Source: CAD feature listing. Evaluate the final solid. Frame: model axes, mm. Face numbers are marked on the shaded views. A direction names the side the tool comes from. Round coordinates to 2 decimals unless told otherwise and drop trailing zeros. Order: outer loops, then holes, each group sorted by start corner. A loop starts at its lowest first (then second) coordinate and runs counter-clockwise, first axis right, second up. Notation, with made-up numbers: (-13.75, 80) - (42.25, 80) arc R33 ccw to (42.25, 115) - close; hole circle Ø11 at (46.5, -8). An arc over 180 degrees is marked (long way). Return JSON: item names as keys, results as strings. Group by question number.
1) Section A-A, the plane z = 11.5. Return loops of the section in (x, y), plus the area to 3 significant figures.
2) Access query for the marked faces 3 and 4. Directions: +Z, -Z, +X, -X, +Y, -Y. A direction counts if a zero-diameter tool reaches every point of the face in a straight line with its end or side. Return the directions, or none.
3) Ray query, line 1 (X direction, y = 2, z = 17); line 2 (Z direction, x = -0.5, y = 4); line 3 (Z direction, x = 0.5, y = 0.5). Return the intervals inside material, ascending. Write a range as from..to.
4) Contact query for flat-ended pins moving along their axis: P1, Ø0.9, axis at x = 0, y = 0.5, coming from the +Z side; P2, Ø1, axis at y = -1, z = 26, coming from the -X side; P3, Ø1, axis at y = 0, z = 18, coming from the +X side. Output: stop coordinate, or through.
5) Mould query, pull axis X, two halves, no side actions, for the marked faces 1 and 2. Classes: pulls with the +X half, pulls with the -X half, needs draft (parallel to the pull), parting line crosses it, or undercut.
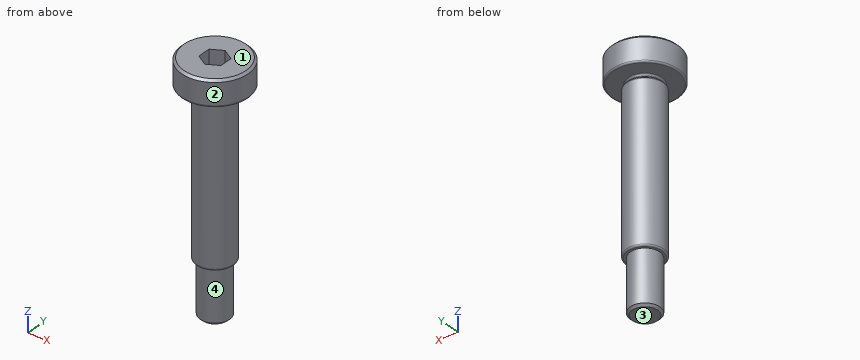
Solid Edge part; units mm, degrees
sketch "Sketch1" plane through (0, 0, 0) normal (0, -1, 0) x (1, 0, 0)
  line L0 (0, 32.7) -> (4.505, 32.7)
  line L1 (4.505, 32.7) -> (4.505, 29.25)
  line L2 (4.505, 29.25) -> (2.1, 29.25)
  line L3 (2.1, 29.25) -> (2.1, 28.85)
  line L4 (2.1, 28.85) -> (2.5, 28.85)
  line L5 (2.5, 28.85) -> (2.5, 7.25)
  line L6 (2.5, 7.25) -> (2, 7.25)
  line L7 (2, 7.25) -> (2, 0)
  line L8 (2, 0) -> (0, 0)
  dimension "D1" = 4.505
  dimension "D2" = 2.1
  dimension "D3" = 2
  dimension "D4" = 2.5
  dimension "D5" = 2
revolve "RevolvedProtrusion1" add sketch "Sketch1" angle 360 about axis through (0, 0, 0) along (0, 0, 1)
chamfer "Chamfer1" distance 0.3 angle 45 3 edges at (-2.5, 0, 28.85) (-4.505, 0, 32.7) (-2, 0, 0)
fillet "Round_1" radius 0.2 4 edges at (-4.505, 0, 29.25) (-2.1, 0, 29.25) (-2.5, 0, 7.25) (-2.5, 0, 28.55)
sketch "Sketch2" plane through (0, 0, 32.7) normal (0, 0, 1) x (1, 0, 0)
  line L0 (1.5, 0.866) -> (0, 1.7321)
  line L1 (0, 1.7321) -> (-1.5, 0.866)
  line L2 (-1.5, 0.866) -> (-1.5, -0.866)
  line L3 (-1.5, -0.866) -> (0, -1.7321)
  line L4 (0, -1.7321) -> (1.5, -0.866)
  line L5 (1.5, -0.866) -> (1.5, 0.866)
extrude "ExtrudedCutout_1" cut sketch "Sketch2" against normal blind 2.4
properties material "Stainless Steel, 304"
Geometry check:
{
 "1": {"outline": "circle Ø5 at (0, 0)", "area": "19.6 mm2"},
 "2": {"face 3": "-Z, +X, -X, +Y, -Y", "face 4": "-Z"},
 "3": {"line 1": "-1.5..1.5", "line 2": "29.25..32.7", "line 3": "0..30.3"},
 "4": {"P1": "z = 30.3", "P2": "x = -2.45", "P3": "x = 2.5"},
 "5": {"face 1": "needs draft", "face 2": "parting line crosses it"}
}
